```python
from build123d import *

# Parameters (mm, degrees)
F0_W     = 58
F0_H     = 58
F0_W_2   = 15
F0_H_2   = 15
F0_R     = 7.5
F1_DEPTH = 1.5
F2_W     = 63
F2_H     = 63
F2_W_2   = 58
F2_H_2   = 58
F3_DEPTH = 15
F4_SIZE2 = 1.2124355653
F4_SIZE  = 0.7
F5_SIZE2 = 5
F5_SIZE  = 1
F6_R     = 2.971748634
F7_DEPTH = 0.5


# Not quite as in the source:
# - a feature names something its author has since deleted; it is built from what else it names


with BuildPart() as f1:
    # F0 (on Top) → F1 (new body)
    with BuildSketch(Plane.XY):
        Rectangle(F0_W, F0_H)
        with Locations((-19, -19)):
            Rectangle(F0_W_2, F0_H_2, mode=Mode.SUBTRACT)
        with Locations((0, -19)):
            Rectangle(F0_W_2, F0_H_2, mode=Mode.SUBTRACT)
        with Locations((19, -19)):
            Rectangle(F0_W_2, F0_H_2, mode=Mode.SUBTRACT)
        with Locations((-19, 0)):
            Rectangle(F0_W_2, F0_H_2, mode=Mode.SUBTRACT)
        with Locations((-19, 19)):
            Circle(F0_R, mode=Mode.SUBTRACT)
        Circle(F0_R, mode=Mode.SUBTRACT)
        with Locations((19, 0)):
            Rectangle(F0_W_2, F0_H_2, mode=Mode.SUBTRACT)
        with Locations((0, 19)):
            Rectangle(F0_W_2, F0_H_2, mode=Mode.SUBTRACT)
        with Locations((19, 19)):
            Rectangle(F0_W_2, F0_H_2, mode=Mode.SUBTRACT)
    extrude(amount=F1_DEPTH)

    # F2 (on Top) → F3 (join)
    with BuildSketch(Plane.XY):
        Rectangle(F2_W, F2_H)
        Rectangle(F2_W_2, F2_H_2, mode=Mode.SUBTRACT)
    extrude(amount=F3_DEPTH)

    # F4
    f4_edges = [f1.edges().sort_by_distance(p)[0] for p in [
        (-26.5, 19, 0),
        (-7.5, 0, 0),
        (-11.5, 0, 0),
        (-19, 7.5, 0),
        (-26.5, 0, 0),
        (-19, -7.5, 0),
        (-19, -11.5, 0),
        (-11.5, -19, 0),
        (-26.5, -19, 0),
        (-19, -26.5, 0),
        (0, -26.5, 0),
        (-7.5, -19, 0),
        (0, -11.5, 0),
        (7.5, -19, 0),
        (11.5, -19, 0),
        (19, -11.5, 0),
        (26.5, -19, 0),
        (19, -26.5, 0),
        (19, -7.5, 0),
        (11.5, 0, 0),
        (19, 7.5, 0),
        (26.5, 0, 0),
        (19, 11.5, 0),
        (11.5, 19, 0),
        (19, 26.5, 0),
        (26.5, 19, 0),
        (7.5, 19, 0),
        (0, 11.5, 0),
        (-7.5, 19, 0),
        (0, 26.5, 0),
    ]]
    chamfer(f4_edges, length=F4_SIZE, length2=F4_SIZE2)

    # F5
    f5_edges = [f1.edges().sort_by_distance(p)[0] for p in [
        (-29, 0, 15),
        (0, 29, 15),
        (29, 0, 15),
        (0, -29, 15),
    ]]
    f5_side = f1.faces().sort_by_distance((0, -30.609045, 15))[0]
    chamfer(f5_edges, length=F5_SIZE, length2=F5_SIZE2, reference=f5_side)

    # F6 (on face) → F7 (cut)
    with BuildSketch(Plane.YZ.offset(31.5)):
        with Locations((0, 7.3488471098)):
            Circle(F6_R)
    extrude(amount=-F7_DEPTH, mode=Mode.SUBTRACT)


solid = f1.part
```
CAD build for the part. Positions are in the model's coordinates, mm. A direction names the side the tool comes from. Coordinates: 2 decimals unless noted, no trailing zeros. Write each loop counter-clockwise with the first axis right and the second up, starting at its lowest first coordinate (ties: lowest second). Pieces come first, ordered by that corner, then holes.
(1) Cut at B-B, the plane y = 0. Count the separate pieces of the cut face and the enclosed holes in it, and give its area (3 significant figures).
(2) Drill centre lines: probe 1 along Y at (x, z) = (0, 1.35); probe 2 along Y at (x, z) = (13.5, 6); probe 3 along X at (y, z) = (0.5, 6.5). Where is each one in solid material? Low to high.
(3) 3-axis set-ups, long thin cutter, end or side, ignore diameter. For faces 5 (the face through (31.254, -0.387, 10.295)), 6 (the face through (0, 29, 6)), 7 (the face through (31.5, 0, 4)): which of +Z, -Z, +X, -X, +Y, -Y reach the whole face in a straight line?
(4) Two-plate mould, pull along Z, no slides. Class faces 1 (the face through (7, 7, 0)), 2 (the face through (-2.5, -30.2, 15)), 3 (the face through (0, -29, 6)), 4 (the face through (31, 0, 7)): +Z half, -Z half, draft (parallel to the pull), parting line (faces both ways), or undercut.
(5) Cut at A-A, the plane x = -19. List the corners of the cut face in (y, z).
(6) Flat gauge pin, fed straight in: pin 1 (8 mm diameter, centred on x = -2.5, y = -4.5, fed in from +Z). Where does the tip first touch, or does it go through?
(7) Cut at C-C, the plane z = 11.25. List the corners of the cut face in (x, y), and give its area (3 significant figures).
Geometry says:
1. separate pieces: 4
1. enclosed holes: 0
1. area: 84.0 mm2
2. probe 1: y = -31.5 to -26.5, -11.5 to -7.5, 7.5 to 11.5, 26.5 to 31.5
2. probe 2: y = -31.5 to -29, 29 to 31.5
2. probe 3: x = -31.5 to -29, 29 to 31
3. face 5: +X
3. face 6: +Z
3. face 7: +Z, -Z, +X, +Y, -Y
4. face 1: -Z half
4. face 2: +Z half
4. face 3: draft
4. face 4: undercut
5. outline: (-31.5, 0) - (-27.2, 0) - (-26.5, 1.21) - (-26.5, 1.5) - (-29, 1.5) - (-29, 10) - (-30, 15) - (-31.5, 15) - close; (-11.5, 1.21) - (-10.8, 0) - (-8.2, 0) - (-7.5, 1.21) - (-7.5, 1.5) - (-11.5, 1.5) - close; (7.5, 1.21) - (8.2, 0) - (10.8, 0) - (11.5, 1.21) - (11.5, 1.5) - (7.5, 1.5) - close; (26.5, 1.21) - (27.2, 0) - (31.5, 0) - (31.5, 15) - (30, 15) - (29, 10) - (29, 1.5) - (26.5, 1.5) - close
6. pin 1: stops at z = 1.5
7. outline: (-31.5, -31.5) - (31.5, -31.5) - (31.5, 31.5) - (-31.5, 31.5) - close; hole (-29.25, -29.25) - (29.25, -29.25) - (29.25, 29.25) - (-29.25, 29.25) - close
7. area: 547 mm2
